Check sheet for the modelled part. Datum: model origin and axes. Units: mm. Face numbers are marked on the shaded views. A direction names the side the tool comes from. Give positions to 0.01 mm unless a question says otherwise; leave off trailing zeros. Order: outer loops, then holes, each group sorted by start corner. A loop starts at its lowest first (then second) coordinate and runs counter-clockwise, first axis right, second up. Notation, with made-up numbers: M -7,16 L 21,16 A24 ccw 21,42 Z; hole C 37,8 d2. An arc over 180 degrees is marked long. One line per question, with ' | ' between items. Start each with the question number.
```python
from build123d import *

# Parameters (mm, degrees)
SKETCH_W        = 32
SKETCH_H        = 26
PAD_DEPTH       = 11
POCKET_DEPTH    = 15
POCKET001_DEPTH = 3
CHAMFER_SIZE    = 5


with BuildPart() as part:
    # Sketch → Pad (new body)
    with BuildSketch(Plane.XY):
        Rectangle(SKETCH_W, SKETCH_H)
    extrude(amount=PAD_DEPTH)

    # Sketch001 (on Face6 of Pad) → Pocket (cut)
    with BuildSketch(Plane.XY.offset(11)):
        with BuildLine():
            ThreePointArc((-10, 1.5), (-11.5, 0), (-10, -1.5))
            Line((-10, -1.5), (10, -1.5))
            ThreePointArc((10, -1.5), (11.5, 0), (10, 1.5))
            Line((10, 1.5), (-10, 1.5))
        make_face()
    extrude(amount=-POCKET_DEPTH, mode=Mode.SUBTRACT)

    # Sketch002 (on Face5 of Pocket) → Pocket001 (cut)
    with BuildSketch(Plane.XY.offset(11)):
        with BuildLine():
            ThreePointArc((-10, 2.75), (-12.75, 0), (-10, -2.75))
            Line((-10, -2.75), (10, -2.75))
            ThreePointArc((10, -2.75), (12.75, 0), (10, 2.75))
            Line((10, 2.75), (-10, 2.75))
        make_face()
    extrude(amount=-POCKET001_DEPTH, mode=Mode.SUBTRACT)

    # Chamfer
    chamfer_edges = [part.edges().sort_by_distance(p)[0] for p in [
        (-16, -13, 5.5),
        (16, -13, 5.5),
        (16, 13, 5.5),
        (-16, 13, 5.5),
    ]]
    chamfer(chamfer_edges, length=CHAMFER_SIZE)


solid = part.part
```
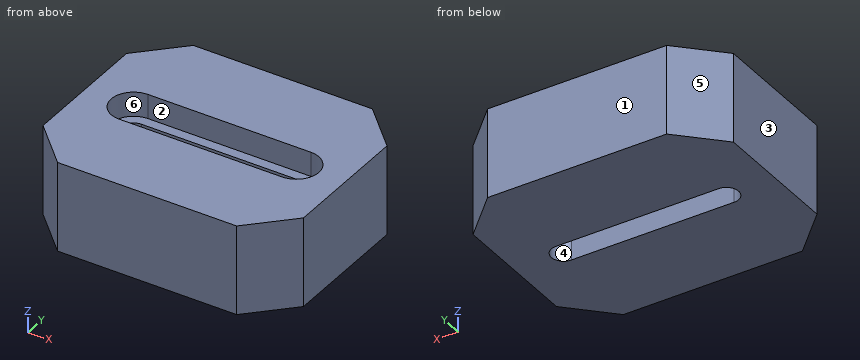
Item 1: Section check D-D, the plane z = 6.5. Record the cut outline in (x, y).
Item 2: Section check B-B, the plane x = 5. Record the cut outline in (y, z).
Item 3: Section check C-C, the plane z = 9.25. Record the cut outline in (x, y), then the cut area to 3 significant figures.
Item 4: Section check A-A, the plane y = 0. Record the cut outline in (x, z).
Item 5: Set-up check for the marked faces 4, 5 and 6: record each of +Z, -Z, +X, -X, +Y, -Y from which the full face is reachable in a straight line by a thin tool's end or side.
Item 6: Go/stop test with a flat-tipped pin: P1, Ø4.5, axis at x = -3.5, y = 0, coming from the +Z side. Record where the tip stops, or that it passes through.
Item 7: Scan lines: probe 1 along Y at (x, z) = (-4.5, 6.75); probe 2 along Y at (x, z) = (7, 9); probe 3 along X at (y, z) = (-11.25, 9.75). Record each from-to range of solid material in increasing order. Write a range as [from, to].
Item 8: Draft check along Y on the marked faces 1, 2 and 3. Enter one of: released by +Y, released by -Y, zero draft, split by the parting line, or undercut.
Reported:
1) outline: M -16,-8 L -11,-13 L 11,-13 L 16,-8 L 16,8 L 11,13 L -11,13 L -16,8 Z; hole M -10,-1.5 L 10,-1.5 A1.5 ccw 10,1.5 L -10,1.5 A1.5 ccw Z
2) outline: M -13,0 L -1.5,0 L -1.5,8 L -2.75,8 L -2.75,11 L -13,11 Z; M 1.5,0 L 13,0 L 13,11 L 2.75,11 L 2.75,8 L 1.5,8 Z
3) outline: M -16,-8 L -11,-13 L 11,-13 L 16,-8 L 16,8 L 11,13 L -11,13 L -16,8 Z; hole M -10,-2.75 L 10,-2.75 A2.75 ccw 10,2.75 L -10,2.75 A2.75 ccw Z | area: 648 mm^2
4) outline: M -16,0 L -11.5,0 L -11.5,8 L -12.75,8 L -12.75,11 L -16,11 Z; M 11.5,0 L 16,0 L 16,11 L 12.75,11 L 12.75,8 L 11.5,8 Z
5) face 4: +Z, -Z | face 5: +Z, -Z, -X, +Y | face 6: +Z
6) P1: stops at z = 8
7) probe 1: y = [-13, -1.5], [1.5, 13] | probe 2: y = [-13, -2.75], [2.75, 13] | probe 3: x = [-12.75, 12.75]
8) face 1: released by +Y | face 2: undercut | face 3: zero draft
